Work out the finished part from the listing and answer in its coordinate system (mm). Face numbers are marked on the shaded views. Give positions to 0.01 mm unless a question says otherwise; leave off trailing zeros. Write each loop counter-clockwise with the first axis right and the second up, starting at its lowest first coordinate (ties: lowest second). Pieces come first, ordered by that corner, then holes. Notation, with made-up numbers: (43.25, 52.25) -> (76.25, 52.25) arc R13 ccw to (76.25, 71.25) -> close; hole circle Ø6 at (-19, 2.25). An arc over 180 degrees is marked (long way). Use a Markdown table: item, result. Add a question column.
Q1. Consider line 1 (Z direction, x = -2.25, y = 0); line 2 (X direction, y = 3, z = -11.25); line 3 (Z direction, x = 2.5, y = -2). Determine where each line is inside the solid, lowest interval first.
Q2. Each of these flat-tipped pins is pushed along its axis until it touches: pin 1 Ø0.9 at (x, y) = (-2, 3) entering from -Z; pin 2 Ø0.9 at (x, z) = (-2, -12) entering from -Y; pin 3 Ø3.5 at (y, z) = (-2, -0.5) entering from +X. Where does it stop, or does it pass through?
Q3. Section D-D, the plane z = -4.5 is taken. Give the vertices of the cut face in (x, y).
Q4. For a pull along Z with two mould halves and no side action, classify the marked faces 1 and 2 as pulls with the +Z half, pulls with the -Z half, needs draft (parallel to the pull), parting line crosses it, or undercut.
Q5. Section B-B, the plane z = -9 is taken. Give the vertices of the cut face in (x, y).
Q6. Section C-C, the plane y = 4 is taken. Give the vertices of the cut face in (x, z).
Q7. Section A-A, the plane y = 0.5 is taken. Give the vertices of the cut face in (x, z).
Autodesk Inventor part; units mm, degrees
ref_plane "РабПлоскость1" through (0, -5, 0) normal (0, 1, 0) x (-1, 0, 0)
ref_plane "РабПлоскость2" through (0, -3, 0) normal (0, 1, 0) x (-1, 0, 0)
ref_plane "YZ Plane" through (0, 0, 0) normal (1, 0, 0) x (0, 1, 0)
sketch "Эскиз1" plane through (0, 0, 0) normal (1, 0, 0) x (0, 1, 0)
  line L0 (-3, -4.5) -> (6, -4.5)
  line L1 (0, -19.9641) -> (0, 3.794)
  line L2 (-7.2118, 0) -> (8.271, 0)
  line L3 (6, -4.5) -> (6, -9.5)
  line L4 (6, -9.5) -> (6, -11.6158) construction
  line L5 (6, -11.6158) -> (2.9383, -13.3469) construction
  line L6 (2.9383, -13.3469) -> (6, -14.7108) construction
  line L7 (6, -14.7108) -> (6, -16.5) construction
  spline S0 degree 4 poles (6, -9.5) (6, -11.6158) (2.9383, -13.3469) (6, -14.7108) (6, -16.5) knots 1 1 1 1 1 2 2 2 2 2
  line L8 (-5, 0) -> (1.5, 0)
  line L9 (3, -1.5) -> (3, -15)
  arc A0 (3, -1.5) -> (1.5, 0) centre (1.5, -1.5) ccw
  point P0 (0, 0)
  dimension "d0" = 9
  dimension "d1" = 3
  dimension "d2" = 4.5
  dimension "d3" = 5
  dimension "d4" = 12
  dimension "d5" = 7
  dimension "d7" = 3
  dimension "d9" = 3
  dimension "d11" = 15
  dimension "d12" = 8
ref_plane "РабПлоскость1" through (0, -5, 0) normal (0, 1, 0) x (-1, 0, 0)
ref_plane "РабПлоскость2" through (0, -3, 0) normal (0, 1, 0) x (-1, 0, 0)
sketch "Эскиз2" plane through (0, -3, 0) normal (0, 1, 0) x (-1, 0, 0)
  line L0 (-3.9, -4) -> (3.9, -4)
  line L1 (3.9, -4) -> (3.9, -5)
  line L2 (3.9, -5) -> (-3.9, -5)
  line L3 (-3.9, -5) -> (-3.9, -4)
  line L4 (0, -5.48) -> (0, 1.38)
  line L5 (0, -4.5) -> (1.03, -4.5)
  point P0 (0, 0)
  dimension "d15" = 7.8
  dimension "d16" = 1
sweep "Сдвиг1" add profiles "Эскиз2" path "Эскиз1" path curves L0 L3 S0
sketch "Эскиз3" plane through (0, -5, 0) normal (0, 1, 0) x (-1, 0, 0)
  line L0 (3.36, 0) -> (-3.36, 0)
  line L1 (0, -0.56) -> (0, 0.56)
  line L2 (2.4, 0.4) -> (1.6, 0.4)
  line L3 (1.6, 0.4) -> (1.6, -0.4)
  line L4 (1.6, -0.4) -> (2.4, -0.4)
  line L5 (2.4, -0.4) -> (2.4, 0.4)
  line L6 (-1.6, 0.4) -> (-2.4, 0.4)
  line L7 (-2.4, 0.4) -> (-2.4, -0.4)
  line L8 (-2.4, -0.4) -> (-1.6, -0.4)
  line L9 (-1.6, -0.4) -> (-1.6, 0.4)
  point P0 (0, 0)
  dimension "d22" = 0.8
  dimension "d23" = 0.8
  dimension "d24" = 0.8
  dimension "d25" = 0.8
  dimension "d26" = 4
sweep "Сдвиг2" add profiles "Эскиз3" path "Эскиз1" path curves L8 A0 L9
sketch "Эскиз4" plane through (0, 0, 0) normal (0, 1, 0) x (-1, 0, 0)
  line L0 (2.4, 0.4) -> (1.6, 0.4)
  line L1 (2.4, -0.4) -> (2.4, 0.4)
  line L2 (1.6, -0.4) -> (2.4, -0.4)
  line L3 (1.6, 0.4) -> (1.6, -0.4)
  line L4 (-1.6, 0.4) -> (-2.4, 0.4)
  line L5 (-1.6, -0.4) -> (-1.6, 0.4)
  line L6 (-2.4, -0.4) -> (-1.6, -0.4)
  line L7 (-2.4, 0.4) -> (-2.4, -0.4)
  line L8 (2.4, 0.4) -> (1.6, 0.4)
  line L9 (1.6, 0.4) -> (1.6, -0.4)
  line L10 (1.6, -0.4) -> (2.4, -0.4)
  line L11 (2.4, -0.4) -> (2.4, 0.4)
  line L12 (-2.4, -0.4) -> (-1.6, -0.4)
  line L13 (-1.6, -0.4) -> (-1.6, 0.4)
  line L14 (-1.6, 0.4) -> (-2.4, 0.4)
  line L15 (-2.4, 0.4) -> (-2.4, -0.4)
  circle A0 centre (-2, 0) radius 0.5657
  point P0 (0, 0)
properties part number "conn_sensor"
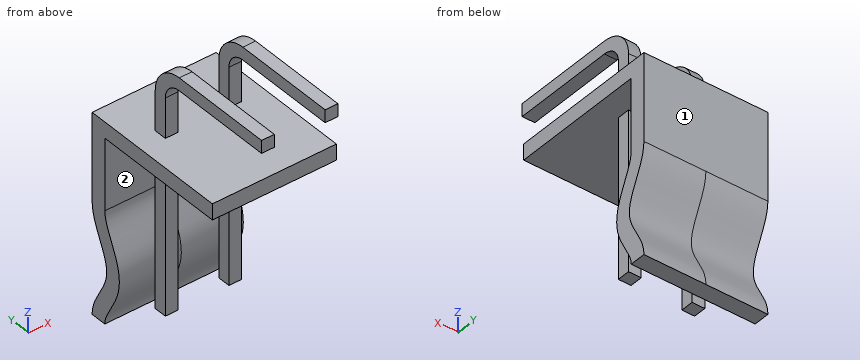
Result set:
| question | item | result |
|---|---|---|
| 1 | line 1 | z = -5 to -4, -0.4 to 0.4 |
| 1 | line 2 | x = -2.4 to -1.6, 1.6 to 2.4 |
| 1 | line 3 | z = -5 to -4 |
| 2 | pin 1 | stops at z = -15 |
| 2 | pin 2 | stops at y = 2.6 |
| 2 | pin 3 | stops at x = 2.4 |
| 3 | outline | (-3.9, -3) -> (3.9, -3) -> (3.9, 6.5) -> (-3.9, 6.5) -> close |
| 4 | face 1 | needs draft |
| 4 | face 2 | undercut |
| 5 | outline | (-3.9, 5.5) -> (3.9, 5.5) -> (3.9, 6.5) -> (-3.9, 6.5) -> close; (-2.4, 2.6) -> (-1.6, 2.6) -> (-1.6, 3.4) -> (-2.4, 3.4) -> close; (1.6, 2.6) -> (2.4, 2.6) -> (2.4, 3.4) -> (1.6, 3.4) -> close |
| 6 | outline | (-3.9, -5) -> (3.9, -5) -> (3.9, -4) -> (-3.9, -4) -> close |
| 7 | outline | (-3.9, -5) -> (3.9, -5) -> (3.9, -4) -> (-3.9, -4) -> close; (-2.4, -0.4) -> (-1.6, -0.4) -> (-1.6, 0.4) -> (-2.4, 0.4) -> close; (1.6, -0.4) -> (2.4, -0.4) -> (2.4, 0.4) -> (1.6, 0.4) -> close |
